```python
from build123d import *

# Parameters (mm, degrees)
F1_DEPTH = 63.5
F0_W     = 25.4
F0_H     = 19.05
F2_DEPTH = 25.4
F3_DEPTH = 7.9375


with BuildPart() as f1:
    # F0 (on Front) → F1 (new body, symmetric)
    with BuildSketch(Plane.XZ):
        Polygon((-41.275, -9.525), (41.275, -9.525), (41.275, 9.525), (22.225, 9.525), (-41.275, 9.525), align=None)
    extrude(amount=F1_DEPTH, both=True)

    # F0 (on Front) → F2 (join, symmetric)
    with BuildSketch(Plane.XZ):
        with BuildLine():
            Line((22.225, 9.525), (41.275, 9.525))
            Line((41.275, 9.525), (41.275, 26.9875))
            ThreePointArc((41.275, 26.9875), (45.9246798487, 38.2128201513), (57.15, 42.8625))
            Line((57.15, 42.8625), (60.325, 42.8625))
            Line((60.325, 42.8625), (60.325, 61.9125))
            Line((60.325, 61.9125), (57.15, 61.9125))
            add(Edge.make_bspline(
                [(55.1065557691, 61.8526683013), (55.7974191484, 61.8796491304), (56.4787770702, 61.8996113569), (57.15, 61.9125)],
                knots=[109.3708422168, 109.3708422168, 109.3708422168, 109.3708422168, 111.4985685166, 111.4985685166, 111.4985685166, 111.4985685166], degree=3))
            ThreePointArc((55.1065557691, 61.8526683013), (31.7420985246, 50.9498489587), (22.225, 26.9875))
            Line((22.225, 26.9875), (22.225, 9.525))
        make_face()
        with Locations((73.025, 52.3875)):
            Rectangle(F0_W, F0_H)
    extrude(amount=F2_DEPTH, both=True)

    # F0 (on Front) → F3 (join, symmetric)
    with BuildSketch(Plane.XZ):
        with BuildLine():
            add(Edge.make_bspline(
                [(-41.275, 9.525), (-41.0335689885, 40.5340906576), (19.5943239296, 60.4657812745), (55.1065557691, 61.8526683013)],
                knots=[0, 0, 0, 0, 109.3708422168, 109.3708422168, 109.3708422168, 109.3708422168], degree=3))
            Line((-41.275, 9.525), (22.225, 9.525))
            Line((22.225, 9.525), (22.225, 26.9875))
            ThreePointArc((22.225, 26.9875), (31.7420985246, 50.9498489587), (55.1065557691, 61.8526683013))
        make_face()
    extrude(amount=F3_DEPTH, both=True)

    # F0 (on Front) → F4 (revolve)
    with BuildSketch(Plane.XZ):
        Polygon((85.725, 61.9125), (85.725, 42.8625), (85.725, 38.1), (111.125, 38.1), (111.125, 66.675), (85.725, 66.675), align=None)
    revolve(axis=Axis((85.725, 0, 52.3875), (0, 0, 1)))


solid = f1.part
```
Geometry: final body of the model. Coordinates: model frame, mm. A direction names the side the tool comes from. Round coordinates to 2 decimals unless told otherwise and drop trailing zeros. Order: outer loops, then holes, each group sorted by start corner. A loop starts at its lowest first (then second) coordinate and runs counter-clockwise, first axis right, second up. Notation, with made-up numbers: M 64.25,-8.5 L 109.25,-8.5 A24 ccw 109.25,15.5 Z; hole C 21,50 d11. An arc over 180 degrees is marked long. One line per item, written item: value.
(1) Cut plane A-A (x = 75). Return the cut outline in (y, z) (1 decimal), and give its area (3 significant figures).
Result sheet:
outline: M -25.4,42.9 L -23,42.9 L -23,38.1 L 23,38.1 L 23,42.9 L 25.4,42.9 L 25.4,61.9 L 23,61.9 L 23,66.7 L -23,66.7 L -23,61.9 L -25.4,61.9 Z
area: 1,410 mm2
(2) Line query: probe 1 along Y at (x, z) = (-15.5, 34.5); probe 2 along Z at (x, y) = (28, 51.5) (3 decimals); probe 3 along X at (y, z) = (36, 2) (3 decimals). Output: solid intervals per line, ascending. Write a range as [from, to].
Result sheet:
probe 1: [-7.94, 7.94]
probe 2: [-9.525, 9.525]
probe 3: [-41.275, 41.275]
(3) Pull-direction query (X, two-part tool) for faces 5 (the flat face through (60, 2, 42.862)), 6 (the flat face through (41.275, -1, 4)), 7 (the flat face through (22.225, -17, 18)); classes: pulls with the +X half, pulls with the -X half, needs draft (parallel to the pull), parting line crosses it, or undercut.
Result sheet:
face 5: undercut
face 6: pulls with the +X half
face 7: pulls with the -X half
(4) Cut plane B-B (z = 4.5). Return the cut outline in (x, y) (3 decimals).
Result sheet:
outline: M -41.275,-63.5 L 41.275,-63.5 L 41.275,63.5 L -41.275,63.5 Z
(5) Cut plane C-C (y = 52). Return the cut outline in (x, z) (3 decimals), and give its area (3 significant figures).
Result sheet:
outline: M -41.275,-9.525 L 41.275,-9.525 L 41.275,9.525 L -41.275,9.525 Z
area: 1,570 mm2
(6) Reachability of faces 1 (the cylindrical face through (32, 16.55, 51.22)), 2 (the cylindrical face through (45.802, -0.356, 38.089)), 3 (the cylindrical face through (32, -16.79, 51.22)), 4 (the flat face through (60, -2, 61.912)) from +Z, -Z, +X, -X, +Y, -Y: full face, straight path, thin tool, end or side. Return the list, or none.
Result sheet:
face 1: +Z, -X, +Y
face 2: -Z, +Y, -Y
face 3: +Z, -X, -Y
face 4: +Z, -X
(7) Pin query (flat end, axial travel): P1, Ø15.5, axis at x = 67, z = 42, coming from the +Y side; P2, Ø11, axis at y = 12.5, z = 0, coming from the +X side (3 decimals); P3, Ø15.5, axis at x = 61.5, z = 42.5, coming from the -Y side. Return the tip coordinate at first contact, or that it passes through.
Result sheet:
P1: y = 25.4
P2: x = 41.275
P3: y = -25.4
